Build history of the part. All positions in model axes, mm. A direction names the side the tool comes from. Give positions to 0.01 mm unless a question says otherwise; leave off trailing zeros. Order: outer loops, then holes, each group sorted by start corner. A loop starts at its lowest first (then second) coordinate and runs counter-clockwise, first axis right, second up. Notation, with made-up numbers: (48, 17.25) - (103, 17.25) arc R12 cw to (103, 38.25) - close; hole circle Ø7 at (42, 85.5). An arc over 180 degrees is marked (long way). Write each question's results on one line, items separated by ' | '. Start each with the question number.
1) Drill centre lines: line 1 along X through (y, z) = (2, 39); line 2 along Z through (x, y) = (120, 2.75); line 3 along X through (y, z) = (-0.5, 37). Where is each one in solid material? Low to high. Write a range as from..to.
2) Tool access for faces 1 (the face through (-64.5, 0.1, 38.9)), 2 (the face through (-8, 11, 40)), 3 (the face through (-12, -11, 40)): list every direction of +Z, -Z, +X, -X, +Y, -Y with a clear straight run to the whole face (end or side of a thin tool).
3) Cut at D-D on x = 58. List the corners of the cut face in (y, z), plus the area to 3 significant figures.
4) Cut at A-A on z = 39. List the corners of the cut face in (x, y).
5) Cut at C-C on y = -8. List the corners of the cut face in (x, z).
6) Two-plate mould, pull along Z, no slides. Class faces 4 (the face through (29, -4.5, 39)), 5 (the face through (-10, 14, 41)), 6 (the face through (117.615, -0.063, 38.249)): +Z half, -Z half, draft (parallel to the pull), parting line (faces both ways), or undercut.
7) Cut at B-B on x = -10. List the corners of the cut face in (y, z).
8) Drop flat-ended pins along their axis: pin 1 Ø2.5 at (x, z) = (-9.5, 37.5) entering from -Y; pin 2 Ø2 at (x, z) = (104.5, 39.5) entering from +Y; pin 3 Ø8 at (x, y) = (-11, -11.5) entering from -Z; pin 4 Ø4 at (x, z) = (120, 39) entering from +Y. Give the stop position or say it passes through.
from build123d import *

# Parameters (mm, degrees)
BOSS_EXTRUDE1_DEPTH          = 9
SKETCH2_R                    = 4
BOSS_EXTRUDE2_DEPTH          = 6.5
BOSS_EXTRUDE4_START          = 6.5
SKETCH4_R                    = 4
BOSS_EXTRUDE4_DEPTH          = 6.5
F_5_0_5_DIAMETER_HOLE1_D     = 5
F_5_0_5_DIAMETER_HOLE1_DEPTH = 23


# Read off the part's stored shape, not the designer's step: Boss-Extrude3, Boss-Extrude5
with BuildPart() as part:
    # Sketch1 → Boss-Extrude1 (new body)
    with BuildSketch(Plane(origin=(0, 4.5, 0), x_dir=(1, 0, 0), z_dir=(0, 1, 0))):
        with BuildLine():
            Line((-60, -43.5), (120, -43.5))
            ThreePointArc((120, -43.5), (124.5, -39), (120, -34.5))
            Line((120, -34.5), (-60, -34.5))
            ThreePointArc((-60, -34.5), (-64.5, -39), (-60, -43.5))
        make_face()
    extrude(amount=-BOSS_EXTRUDE1_DEPTH)

    # Sketch2 → Boss-Extrude2 (add)
    with BuildSketch(Plane.XZ.offset(4.5)):
        with Locations(Location((-10, 39, 0), (0, 0, 90))):
            Circle(SKETCH2_R)
    extrude(amount=BOSS_EXTRUDE2_DEPTH)

    # Boss-Extrude3 outline → Boss-Extrude3 (revolve)
    with BuildSketch(Plane(origin=(-10, 0, 39), x_dir=(1, 0, 0), z_dir=(0, 0, 1))):
        with BuildLine():
            ThreePointArc((0, -18.5), (1.414213563, -17.914213562), (2, -16.499999998))
            Line((2, -16.499999998), (2, -11))
            Line((2, -11), (0, -11))
            Line((0, -11), (0, -18.5))
        make_face()
    revolve(axis=Axis((-10, 0, 39), (0, 1, 0)))

    # Sketch4 → Boss-Extrude4 (add)
    with BuildSketch(Plane(origin=(0, 4.5, 0), x_dir=(-1, 0, 0), z_dir=(0, 1, 0)).offset(BOSS_EXTRUDE4_START)):
        with Locations(Location((10, 39, 0), (0, 0, 90))):
            Circle(SKETCH4_R)
    extrude(amount=-BOSS_EXTRUDE4_DEPTH)

    # Boss-Extrude5 outline → Boss-Extrude5 (revolve)
    with BuildSketch(Plane(origin=(-10, 0, 39), x_dir=(1, 0, 0), z_dir=(0, 0, 1))):
        with BuildLine():
            Line((2, 11), (2, 16.499999998))
            ThreePointArc((2, 16.499999998), (1.414213563, 17.914213562), (0, 18.5))
            Line((0, 18.5), (0, 11))
            Line((0, 11), (2, 11))
        make_face()
    revolve(axis=Axis((-10, 0, 39), (0, 1, 0)))

    # Ø5.0 (5) Diameter Hole1
    with Locations(Plane(origin=(0, 4.5, 0), x_dir=(1, 0, 0), z_dir=(0, 1, 0))):
        with Locations((-60, -39), (120, -39)):
            Hole(F_5_0_5_DIAMETER_HOLE1_D / 2, depth=F_5_0_5_DIAMETER_HOLE1_DEPTH)


solid = part.part
Results:
1) line 1: -64.5..-62.5, -57.5..117.5, 122.5..124.5 | line 2: 34.5..36.5, 41.5..43.5 | line 3: -64.03..-61.5, -58.5..118.5, 121.5..124.03
2) face 1: -X, +Y, -Y | face 2: +Y | face 3: -Y
3) outline: (-4.5, 34.5) - (4.5, 34.5) - (4.5, 43.5) - (-4.5, 43.5) - close | area: 81.0 mm^2
4) outline: (-64.5, -4.5) - (-62.5, -4.5) - (-62.5, 4.5) - (-64.5, 4.5) - close; (-57.5, -4.5) - (-14, -4.5) - (-14, -11) - (-12, -11) - (-12, -16.5) arc R2 ccw to (-8, -16.5) - (-8, -11) - (-6, -11) - (-6, -4.5) - (117.5, -4.5) - (117.5, 4.5) - (-6, 4.5) - (-6, 11) - (-8, 11) - (-8, 16.5) arc R2 ccw to (-12, 16.5) - (-12, 11) - (-14, 11) - (-14, 4.5) - (-57.5, 4.5) - close; (122.5, -4.5) - (124.5, -4.5) - (124.5, 4.5) - (122.5, 4.5) - close
5) outline: circle Ø8 at (-10, 39)
6) face 4: draft | face 5: parting line | face 6: undercut
7) outline: (-16.5, 37) - (-11, 37) - (-11, 35) - (-4.5, 35) - (-4.5, 34.5) - (4.5, 34.5) - (4.5, 35) - (11, 35) - (11, 37) - (16.5, 37) arc R2 ccw to (16.5, 41) - (11, 41) - (11, 43) - (4.5, 43) - (4.5, 43.5) - (-4.5, 43.5) - (-4.5, 43) - (-11, 43) - (-11, 41) - (-16.5, 41) arc R2 ccw to start
8) pin 1: y = -18.47 | pin 2: y = 4.5 | pin 3: z = 35 | pin 4: through
